Input: part model. Units: mm. Frame: model coordinates. A direction names the side the tool comes from. Round coordinates to 2 decimals unless told otherwise and drop trailing zeros. Loops run counter-clockwise (first coordinate to the right, second up) from the corner with the lowest first, then second, coordinate; pieces in that order, holes last. Notation, with made-up numbers: M 28.25,80.5 L 63.25,80.5 A22 cw 63.25,115.5 Z; hole C 38,-16.75 d1. An arc over 180 degrees is marked long. Put each result on its own line as item: value. Start each with the question number.
1) Section B-B on z = 34.5. Output: boundary loops of the cut face in (x, y).
2) Section C-C on z = 5. Output: boundary loops of the cut face in (x, y), plus the area to 3 significant figures.
3) Pin query (flat end, axial travel): pin 1 (4 mm diameter, centred on y = 104.5, z = 28, fed in from +X); pin 2 (10 mm diameter, centred on x = 92.11, z = 23.81, fed in from +Y); pin 3 (1.5 mm diameter, centred on x = 101, z = 33, fed in from -Y). Return the tip coordinate at first contact, or that it passes through.
4) Reachability of faces 5 (the face through (73, 60.385, 23)), 6 (the face through (96, 93.71, 23)), 7 (the face through (106.77, 85.41, 23.48)) from +Z, -Z, +X, -X, +Y, -Y: full face, straight path, thin tool, end or side. Return the list, or none.
5) Section A-A on y = 64. Output: boundary loops of the cut face in (x, z) (3 decimals), plus the area to 3 significant figures.
6) Draft query along Z for faces 1 (the face through (77.41, 85.35, 23.48)), 2 (the face through (89, 89, 0)), 3 (the face through (89, 89, 47.625)), 4 (the face through (75.4, 98.56, 10.42)). Return one class per face: +Z half, -Z half, draft (parallel to the pull), parting line (faces both ways), or undercut.
7) Line query: probe 1 along X at (y, z) = (77.5, 17); probe 2 along X at (y, z) = (104, 31.5); probe 3 along Y at (x, z) = (91, 30). Output: solid intervals per line, ascending.
from build123d import *

# Parameters (mm, degrees)
BOSS_EXTRUDE2_DEPTH = 47.625
SKETCH2_R           = 3.175
CUT_EXTRUDE1_DEPTH  = 127.847111609
SKETCH4_R           = 3.175
CUT_EXTRUDE2_DEPTH  = 128.089653795
SKETCH5_R           = 3.175
CUT_EXTRUDE3_DEPTH  = 47.625


with BuildPart() as part:
    # Model → Boss-Extrude2 (new body)
    with BuildSketch(Plane.XY):
        Polygon((112.745318321, 60.38539613), (112.745318321, 93.710196132), (79.420518319, 93.710196132), (79.420518319, 110.37259613), (71.49571832, 110.37259613), (71.49571832, 60.38539613), (75.45811832, 60.38539613), (75.45811832, 83.397796131), (79.420518319, 87.360196131), (104.82051832, 87.360196131), (108.782918319, 83.397796131), (108.782918319, 60.38539613), align=None)
    extrude(amount=BOSS_EXTRUDE2_DEPTH)

    # Sketch2 → Cut-Extrude1 (cut, through all)
    with BuildSketch(Plane(origin=(0, 93.710196132, 0), x_dir=(1, 0, 0), z_dir=(0, 1, 0))):
        with Locations(Location((92.107818321, -23.8125, 0), (0, 0, 270))):
            Circle(SKETCH2_R)
    extrude(amount=-CUT_EXTRUDE1_DEPTH, mode=Mode.SUBTRACT)

    # Sketch4 → Cut-Extrude2 (cut, through all)
    with BuildSketch(Plane.ZY.offset(-71.49571832)):
        with Locations((11.1125, 101.66039613)):
            Circle(SKETCH4_R)
        with Locations((36.5125, 101.66039613)):
            Circle(SKETCH4_R)
    extrude(amount=-CUT_EXTRUDE2_DEPTH, mode=Mode.SUBTRACT)

    # Sketch5 → Cut-Extrude3 (cut)
    with BuildSketch(Plane(origin=(112.745318321, 0, 0), x_dir=(0, 0, -1), z_dir=(1, 0, 0))):
        with Locations((-23.8125, 69.91039613)):
            Circle(SKETCH5_R)
    extrude(amount=-CUT_EXTRUDE3_DEPTH, mode=Mode.SUBTRACT)


solid = part.part
Geometry results:
1. outline: M 71.5,60.39 L 75.46,60.39 L 75.46,83.4 L 79.42,87.36 L 104.82,87.36 L 108.78,83.4 L 108.78,60.39 L 112.75,60.39 L 112.75,93.71 L 79.42,93.71 L 79.42,99.2 L 71.5,99.2 Z; M 71.5,104.12 L 79.42,104.12 L 79.42,110.37 L 71.5,110.37 Z
2. outline: M 71.5,60.39 L 75.46,60.39 L 75.46,83.4 L 79.42,87.36 L 104.82,87.36 L 108.78,83.4 L 108.78,60.39 L 112.75,60.39 L 112.75,93.71 L 79.42,93.71 L 79.42,110.37 L 71.5,110.37 Z
2. area: 623 mm²
3. pin 1: stops at x = 79.42
3. pin 2: stops at y = 93.71
3. pin 3: stops at y = 87.36
4. face 5: +Z, -Z, +X, -X, -Y
4. face 6: +Z, -Z, +X, +Y
4. face 7: +Z, -Z, -Y
5. outline: M 71.496,0 L 75.458,0 L 75.458,47.625 L 71.496,47.625 Z; M 108.783,0 L 112.745,0 L 112.745,47.625 L 108.783,47.625 Z
5. area: 377 mm²
6. face 1: draft
6. face 2: -Z half
6. face 3: +Z half
6. face 4: undercut
7. probe 1: x = 71.5 to 75.46, 108.78 to 112.75
7. probe 2: x = 71.5 to 79.42
7. probe 3: y = 87.36 to 93.71
